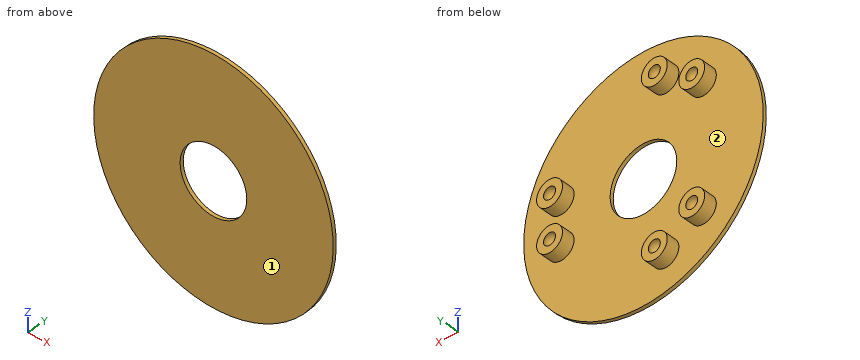
```python
from build123d import *

# Parameters (mm, degrees)
SKETCH1_R          = 692.820324
SKETCH1_R_2        = 192.820324
EXTRUDE1_DEPTH     = 20
SKETCH2_R          = 75
CUT_EXTRUDE1_DEPTH = 10


# Read off the part's stored shape, not the designer's step: 连接重组1
with BuildPart() as part:
    # Sketch1 → Extrude1 (new body)
    with BuildSketch(Plane(origin=(0, 0, 0), x_dir=(1, 0, 0), z_dir=(0, 1, 0))):
        with Locations(Location((0, 0, 0), (0, 0, 270))):
            Circle(SKETCH1_R)
        with Locations(Location((0, 0, 0), (0, 0, 270))):
            Circle(SKETCH1_R_2, mode=Mode.SUBTRACT)
    extrude(amount=-EXTRUDE1_DEPTH)

    # Sketch2 → Cut-Extrude1 (cut)
    with BuildSketch(Plane(origin=(0, 0, 0), x_dir=(1, 0, 0), z_dir=(0, 1, 0))):
        with Locations(Location((-129.90381057, 475, 0), (0, 0, 270))):
            Circle(SKETCH2_R)
        with Locations(Location((-129.90381057, -475, 0), (0, 0, 270))):
            Circle(SKETCH2_R)
        with Locations(Location((476.314, -125, 0), (0, 0, 270))):
            Circle(SKETCH2_R)
        with Locations(Location((-346.4101615, 350, 0), (0, 0, 270))):
            Circle(SKETCH2_R)
        with Locations(Location((-346.4101615, -350, 0), (0, 0, 270))):
            Circle(SKETCH2_R)
        with Locations(Location((476.314, 125, 0), (0, 0, 270))):
            Circle(SKETCH2_R)
    extrude(amount=-CUT_EXTRUDE1_DEPTH, mode=Mode.SUBTRACT)

    # 连接重组1 outline → 连接重组1 (revolve)
    with BuildSketch(Plane(origin=(476.314, 0, 125), x_dir=(1, 0, 0), z_dir=(0, 0, 1))):
        with BuildLine():
            Line((75, 75), (34.641016131, 75.000000035))
            ThreePointArc((34.641016131, 75.000000035), (34.641016161, 35.000000018), (0, 15))
            Line((0, 15), (0, -10))
            Line((0, -10), (75, -10))
            Line((75, -10), (75, 75))
        make_face()
    revolve(axis=Axis((476.314, 0, 125), (0, 1, 0)))

    # Other 1 2 outline → Other 1 2 (revolve)
    with BuildSketch(Plane(origin=(-129.90381057, 0, 475), x_dir=(1, 0, 0), z_dir=(0, 0, 1))):
        with BuildLine():
            Line((75, 75), (34.641016131, 75.000000035))
            ThreePointArc((34.641016131, 75.000000035), (34.641016161, 35.000000018), (0, 15))
            Line((0, 15), (0, -10))
            Line((0, -10), (75, -10))
            Line((75, -10), (75, 75))
        make_face()
    revolve(axis=Axis((-129.90381057, 0, 475), (0, 1, 0)))

    # Other 1 3 outline → Other 1 3 (revolve)
    with BuildSketch(Plane(origin=(-346.4101615, 0, -350), x_dir=(1, 0, 0), z_dir=(0, 0, 1))):
        with BuildLine():
            Line((75, 75), (34.641016131, 75.000000035))
            ThreePointArc((34.641016131, 75.000000035), (34.641016161, 35.000000018), (0, 15))
            Line((0, 15), (0, -10))
            Line((0, -10), (75, -10))
            Line((75, -10), (75, 75))
        make_face()
    revolve(axis=Axis((-346.4101615, 0, -350), (0, 1, 0)))

    # Other 1 4 outline → Other 1 4 (revolve)
    with BuildSketch(Plane(origin=(-129.90381057, 0, -475), x_dir=(1, 0, 0), z_dir=(0, 0, 1))):
        with BuildLine():
            Line((75, 75), (34.641016131, 75.000000035))
            ThreePointArc((34.641016131, 75.000000035), (34.641016161, 35.000000018), (0, 15))
            Line((0, 15), (0, -10))
            Line((0, -10), (75, -10))
            Line((75, -10), (75, 75))
        make_face()
    revolve(axis=Axis((-129.90381057, 0, -475), (0, 1, 0)))

    # Other 1 5 outline → Other 1 5 (revolve)
    with BuildSketch(Plane(origin=(-346.4101615, 0, 350), x_dir=(1, 0, 0), z_dir=(0, 0, 1))):
        with BuildLine():
            Line((75, 75), (34.641016131, 75.000000035))
            ThreePointArc((34.641016131, 75.000000035), (34.641016161, 35.000000018), (0, 15))
            Line((0, 15), (0, -10))
            Line((0, -10), (75, -10))
            Line((75, -10), (75, 75))
        make_face()
    revolve(axis=Axis((-346.4101615, 0, 350), (0, 1, 0)))

    # Other 1 6 outline → Other 1 6 (revolve)
    with BuildSketch(Plane(origin=(476.314, 0, -125), x_dir=(1, 0, 0), z_dir=(0, 0, 1))):
        with BuildLine():
            Line((75, 75), (34.641016131, 75.000000035))
            ThreePointArc((34.641016131, 75.000000035), (34.641016161, 35.000000018), (0, 15))
            Line((0, 15), (0, -10))
            Line((0, -10), (75, -10))
            Line((75, -10), (75, 75))
        make_face()
    revolve(axis=Axis((476.314, 0, -125), (0, 1, 0)))


solid = part.part
```
Source: CAD feature listing. Evaluate the final solid. Frame: model axes, mm. Face numbers are marked on the shaded views. Round coordinates to 2 decimals unless told otherwise and drop trailing zeros. Loops run counter-clockwise (first coordinate to the right, second up) from the corner with the lowest first, then second, coordinate; pieces in that order, holes last. Notation, with made-up numbers: M -4.5,-22 L 37.5,-22 A29 cw 37.5,3 Z; hole C 35.5,70.25 d11. An arc over 180 degrees is marked long. Put each result on its own line as item: value.
(1) First-contact query: pin 1 (1 mm diameter, centred on x = 52.5, z = 433.5, fed in from +Y); pin 2 (1 mm diameter, centred on y = -1.5, z = -110.5, fed in from +X); pin 3 (12 mm diameter, centred on y = 33, z = 138.5, fed in from -X); pin 4 (8 mm diameter, centred on x = 307, y = 4.5, fed in from -Z). Flat tips, straight axial feed; report the tip coordinate or a pass-through.
Solutions:
pin 1: y = 0
pin 2: x = 684.03
pin 3: x = 401.69
pin 4: through
(2) Ray query, line 1 (X direction, y = -8, z = 0); line 2 (Z direction, x = -307.5, y = 15); line 3 (Y direction, x = -254, z = 591). Return the intervals inside material, ascending. Write a range as [from, to].
Solutions:
line 1: [-692.82, -192.82], [192.82, 692.82]
line 2: [-414.12, -285.88], [285.88, 414.12]
line 3: [-20, 0]
(3) Section D-D, the plane z = 475. Return loops of the section in (x, y), and give its area (3 significant figures).
Solutions:
outline: M -504.36,-20 L 504.36,-20 L 504.36,0 L -54.9,0 L -54.9,75 L -95.26,75 A40 cw long -164.54,75 L -204.9,75 L -204.9,0 L -504.36,0 Z
area: 27,400 mm²
(4) Section A-A, the plane y = 57. State how many separate pieces and enclosed holes the cut face has, and give its area (3 significant figures).
Solutions:
separate pieces: 6
enclosed holes: 6
area: 75,900 mm²
(5) Pull-direction query (Z, two-part tool) for the marked faces 1 and 2; classes: released by +Z, released by -Z, zero draft, split by the parting line, or undercut.
Solutions:
face 1: zero draft
face 2: undercut
(6) Section C-C, the plane z = 31. Return loops of the section in (x, y).
Solutions:
outline: M -692.13,-20 L -190.31,-20 L -190.31,0 L -692.13,0 Z; M 190.31,-20 L 692.13,-20 L 692.13,0 L 190.31,0 Z
(7) Section B-B, the plane x = 0. Return loops of the section in (y, z), and give its area (3 significant figures).
Solutions:
outline: M -20,-692.82 L 0,-692.82 L 0,-192.82 L -20,-192.82 Z; M -20,192.82 L 0,192.82 L 0,692.82 L -20,692.82 Z
area: 20,000 mm²
